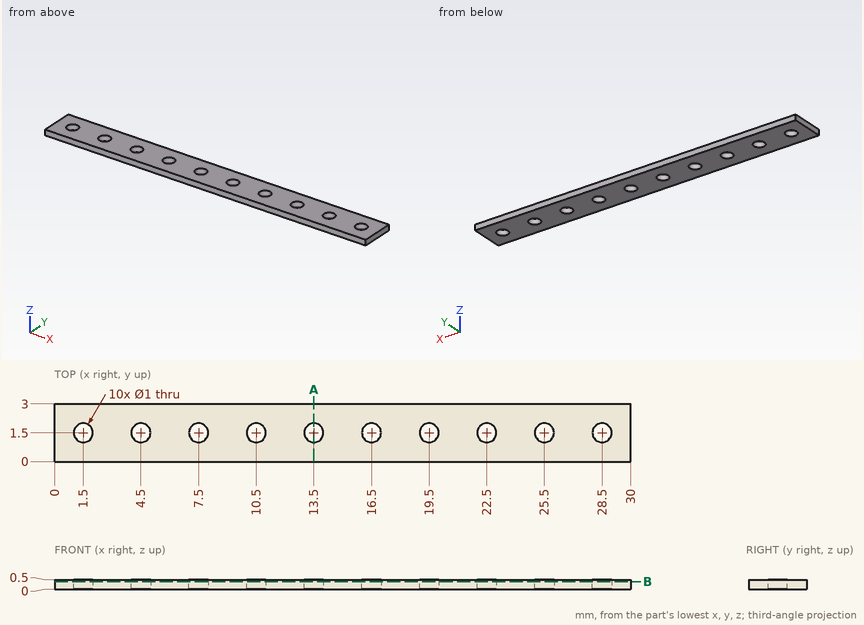
Design review of the part shown in the three views and the two pictorial views. Dimensions are in mm from the part's minimum x, y and z. Round coordinates to 2 decimals unless told otherwise and drop trailing zeros. Loops run counter-clockwise (first coordinate to the right, second up) from the corner with the lowest first, then second, coordinate; pieces in that order, holes last. Notation, with made-up numbers: M 22.5,-28 L 60.5,-28 A18 ccw 60.5,-1 Z; hole C -23.75,18 d3. An arc over 180 degrees is marked long. Answer as a JSON object with one key per item and string values.
Item 1: We need section B-B, the plane z = 0.4. State how many separate pieces and enclosed holes the cut face has, and give its area (3 significant figures).
Check sheet entries:
{"separate pieces": "1", "enclosed holes": "10", "area": "82.1 mm2"}
Item 2: We need section A-A, the plane x = 13.5. State the section outline as (y, z) points, and give its area (3 significant figures).
Check sheet entries:
{"outline": "M 0,0 L 1,0 L 1,0.5 L 0,0.5 Z; M 2,0 L 3,0 L 3,0.5 L 2,0.5 Z", "area": "1.00 mm2"}
Item 3: For line 1 along Y through (x, z) = (25.5, 0.2), list the stretches that pass through material, from the lowest coordinate up.
Check sheet entries:
{"line 1": "0 to 1, 2 to 3"}
